Answer from the drawing. Dimensions are ordinates in mm from the lowest x, y and z of the part. A direction names the side the tool comes from. Give positions to 0.01 mm unless a question says otherwise; leave off trailing zeros. Loops run counter-clockwise (first coordinate to the right, second up) from the corner with the lowest first, then second, coordinate; pieces in that order, holes last. Notation, with made-up numbers: (68.25, 52.5) -> (96.25, 52.5) arc R14 ccw to (96.25, 58.5) -> close; hole circle Ø11 at (73, 71). An arc over 180 degrees is marked (long way). Write each question's results on one line, items separated by ' | '. Start each with the question number.
Item 1: Section C-C on y = 15.5 is taken. Write down the section's boundary in (x, z), and give its area (3 significant figures).
Item 2: Which of the six approach directions +Z, -Z, +X, -X, +Y, -Y give full straight-line access (tool end or side, diameter ignored) to the marked faces 1 and 2?
Item 3: Section D-D on x = 66.5 is taken. Write down the section's boundary in (y, z) (1 decimal).
Item 4: Each of these flat-tipped pins is pushed along its axis until it touches: P1, Ø9, axis at x = 10, y = 61.49, coming from the -Z side; P2, Ø5, axis at x = 51, z = 2, coming from the -Y side; P3, Ø4, axis at x = 134.92, y = 11.3, coming from the -Z side; P4, Ø6, axis at y = 44.5, z = 5, coming from the +X side (1 decimal). Where does it stop, or does it pass through?
Item 5: Find the intervals of material crossed by line 1 (Y direction, x = 10, z = 6.75) (1 decimal); line 2 (Y direction, x = 31.5, z = 4.5); line 3 (X direction, y = 62.5, z = 2.75) (1 decimal), in increasing order.
Item 6: Section B-B on z = 7.25 is taken. Write down the section's boundary in (x, y) (1 decimal).
Item 7: Section A-A on x = 10 is taken. Write down the section's boundary in (y, z) (1 decimal).
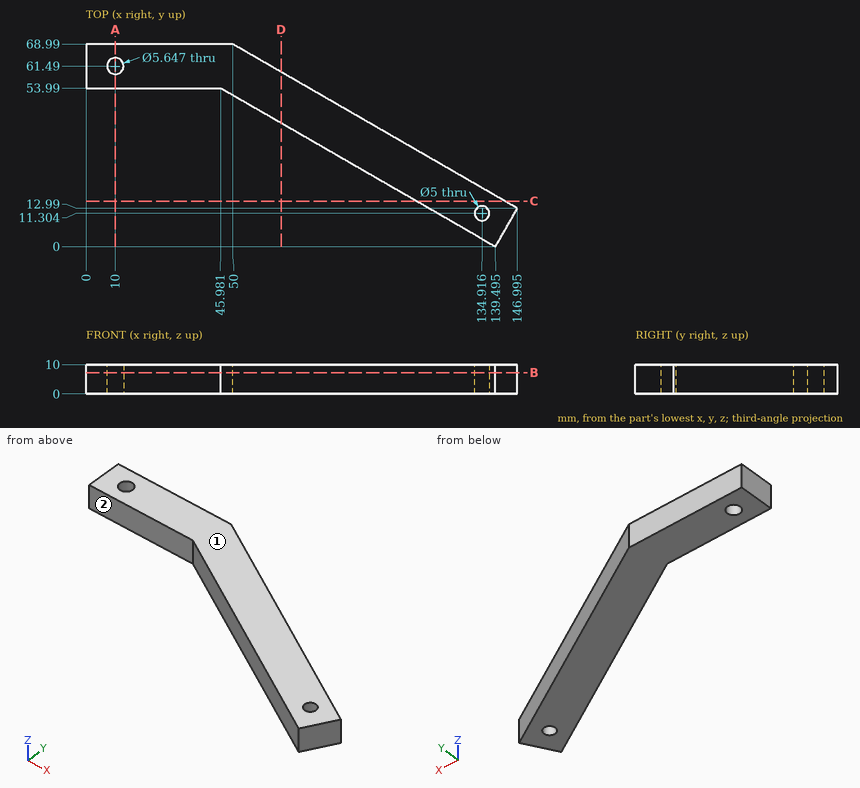
Findings:
1) outline: (112.65, 0) -> (142.65, 0) -> (142.65, 10) -> (112.65, 10) -> close | area: 300 mm2
2) face 1: +Z, +X, -X, +Y, -Y | face 2: +Z, -Z, -X, -Y
3) outline: (42.1, 0) -> (59.5, 0) -> (59.5, 10) -> (42.1, 10) -> close
4) P1: z = 0 | P2: y = 49.65 | P3: through | P4: x = 97.6
5) line 1: 54 to 58.7, 64.3 to 69 | line 2: 53.99 to 68.99 | line 3: 0 to 7.4, 12.6 to 61.2
6) outline: (0, 54) -> (46, 54) -> (139.5, 0) -> (147, 13) -> (50, 69) -> (0, 69) -> close; hole circle Ø5.6 at (10, 61.5); hole circle Ø5 at (134.9, 11.3)
7) outline: (54, 0) -> (58.7, 0) -> (58.7, 10) -> (54, 10) -> close; (64.3, 0) -> (69, 0) -> (69, 10) -> (64.3, 10) -> close
